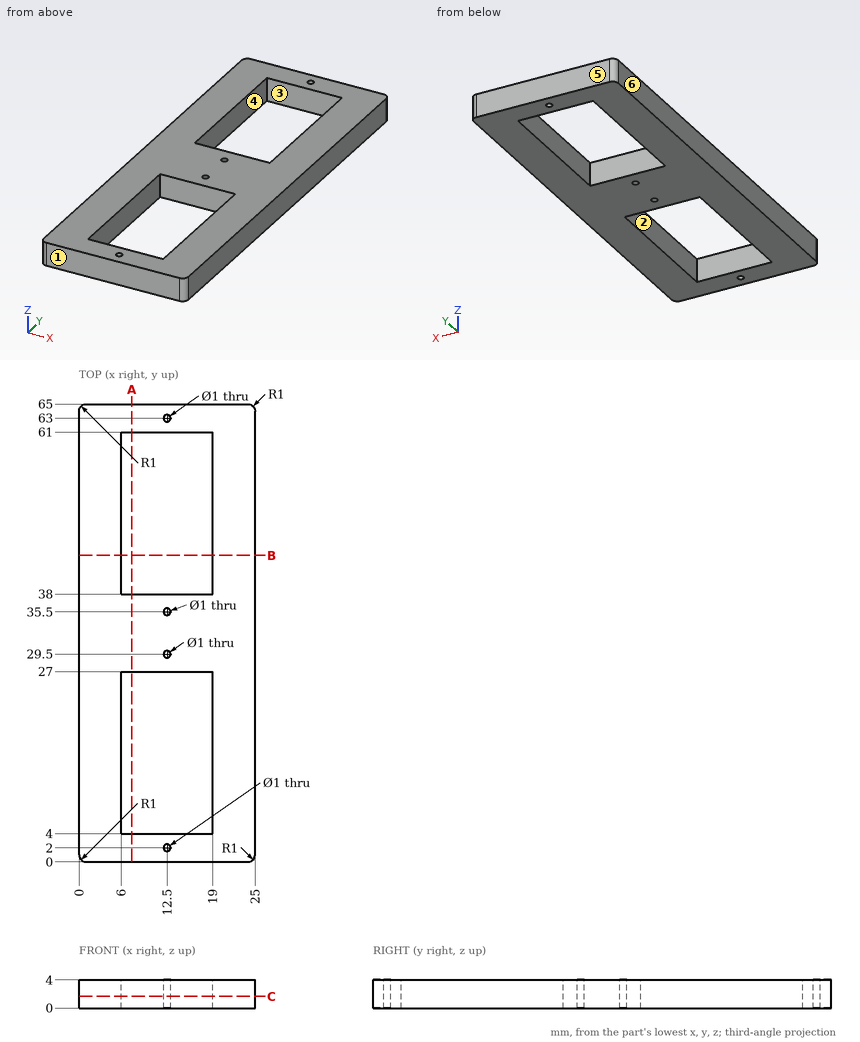
Verification items for this drawing (mm, ordinates from the low corner). A direction names the side the tool comes from. Give positions to 0.01 mm unless a question says otherwise; leave off trailing zeros. Loops run counter-clockwise (first coordinate to the right, second up) from the corner with the lowest first, then second, coordinate; pieces in that order, holes last.
1. Tool access check on the marked faces 1 and 2. Record the directions out of +Z, -Z, +X, -X, +Y, -Y that give a thin tool (end or side, any length) a straight path to the whole face; none if there is none.
Derived:
face 1: +Z, -Z, +X, -X, -Y
face 2: +Z, -Z
2. Material ranges on probe 1 along Y at (x, z) = (13.25, 2.35); probe 2 along X at (y, z) = (49.5, 1); probe 3 along X at (y, z) = (35.5, 2.65), recorded low to high.
Derived:
probe 1: y = 0 to 4, 27 to 38, 61 to 65
probe 2: x = 0 to 6, 19 to 25
probe 3: x = 0 to 12, 13 to 25
3. Release check for a two-part mould opening along X. For the marked faces 3, 4, 5 and 6 record: +X half, -X half, draft (parallel to the pull), parting line (faces both ways), or undercut.
Derived:
face 3: undercut
face 4: undercut
face 5: draft
face 6: -X half
4. Cross-section at A-A on x = 7.5. Record the cut outline in (y, z).
Derived:
outline: (0, 0) - (4, 0) - (4, 4) - (0, 4) - close; (27, 0) - (38, 0) - (38, 4) - (27, 4) - close; (61, 0) - (65, 0) - (65, 4) - (61, 4) - close
5. Cross-section at C-C on z = 1.65. Record the cut outline in (x, y).
Derived:
outline: (0, 1) arc R1 ccw to (1, 0) - (24, 0) arc R1 ccw to (25, 1) - (25, 64) arc R1 ccw to (24, 65) - (1, 65) arc R1 ccw to (0, 64) - close; hole (6, 4) - (19, 4) - (19, 27) - (6, 27) - close; hole (6, 38) - (19, 38) - (19, 61) - (6, 61) - close; hole circle Ø1 at (12.5, 2); hole circle Ø1 at (12.5, 29.5); hole circle Ø1 at (12.5, 35.5); hole circle Ø1 at (12.5, 63)
6. Cross-section at B-B on y = 43.5. Record the cut outline in (x, z).
Derived:
outline: (0, 0) - (6, 0) - (6, 4) - (0, 4) - close; (19, 0) - (25, 0) - (25, 4) - (19, 4) - close
